```python
from build123d import *

# Parameters (mm, degrees)
SKETCH1_W           = 20
SKETCH1_H           = 20
BOSS_EXTRUDE1_DEPTH = 5
CHAMFER1_SIZE       = 3
FILLET1_R           = 3


with BuildPart() as part:
    # Sketch1 → Boss-Extrude1 (new body)
    with BuildSketch(Plane(origin=(0, 0, 0), x_dir=(1, 0, 0), z_dir=(0, 1, 0))):
        with Locations((10, 10)):
            Rectangle(SKETCH1_W, SKETCH1_H)
    extrude(amount=BOSS_EXTRUDE1_DEPTH)

    # Chamfer1
    chamfer1_edges = [part.edges().sort_by_distance(p)[0] for p in [
        (10, 5, -20),
        (0, 5, -10),
        (10, 5, 0),
        (20, 5, -10),
    ]]
    chamfer(chamfer1_edges, length=CHAMFER1_SIZE)

    # Fillet1
    # the kernel refuses this fillet: 3 mm, written as the material it takes off along each edge
    with BuildSketch(Plane(origin=(0, -7.5, 0), x_dir=(0, 0, -1), z_dir=(0, 1, 0)), Plane(origin=(0, -7.5, -20), x_dir=(1, 0, 0), z_dir=(0, 1, 0))) as fillet1_piece_1:
        with BuildLine():
            CenterArc((FILLET1_R, -FILLET1_R), FILLET1_R, 90, 90)
            Line((0, -FILLET1_R), (0, 0))
            Line((0, 0), (FILLET1_R, 0))
        make_face()
    extrude(amount=17, mode=Mode.SUBTRACT)
    with BuildSketch(Plane(origin=(20, -7.5, -20), x_dir=(-1, 0, 0), z_dir=(0, 1, 0)), Plane(origin=(20, -7.5, 0), x_dir=(0, 0, -1), z_dir=(0, 1, 0))) as fillet1_piece_2:
        with BuildLine():
            CenterArc((FILLET1_R, FILLET1_R), FILLET1_R, 180, 90)
            Line((0, FILLET1_R), (0, 0))
            Line((0, 0), (FILLET1_R, 0))
        make_face()
    extrude(amount=17, mode=Mode.SUBTRACT)
    with BuildSketch(Plane(origin=(22.5, -0.5, -22.5), x_dir=(-0.8164965809277263, -0.4082482904638636, -0.408248290463862), z_dir=(-0.5773502691896255, 0.577350269189626, 0.577350269189626)), Plane(origin=(22.5, -0.5, 2.5), x_dir=(0.4082482904638631, -0.4082482904638628, -0.8164965809277261), z_dir=(-0.5773502691896261, 0.5773502691896256, -0.5773502691896256))) as fillet1_piece_3:
        with BuildLine():
            CenterArc((FILLET1_R * 0.57735026919, FILLET1_R), FILLET1_R, 210, 60)
            Line((-FILLET1_R * 0.288675134595, FILLET1_R * 0.5), (0, 0))
            Line((0, 0), (FILLET1_R * 0.57735026919, 0))
        make_face()
    extrude(amount=13.856406461, mode=Mode.SUBTRACT)
    with BuildSketch(Plane(origin=(-2.5, -0.5, -22.5), x_dir=(0.8164965809277259, -0.40824829046386324, -0.40824829046386274), z_dir=(0.5773502691896258, 0.5773502691896258, 0.5773502691896258)), Plane(origin=(-2.5, -0.5, 2.5), x_dir=(-0.40824829046386274, -0.4082482904638633, -0.816496580927726), z_dir=(0.5773502691896258, 0.5773502691896258, -0.5773502691896258))) as fillet1_piece_4:
        with BuildLine():
            CenterArc((FILLET1_R * 0.57735026919, -FILLET1_R), FILLET1_R, 90, 60)
            Line((-FILLET1_R * 0.288675134595, -FILLET1_R * 0.5), (0, 0))
            Line((0, 0), (FILLET1_R * 0.57735026919, 0))
        make_face()
    extrude(amount=13.856406461, mode=Mode.SUBTRACT)


solid = part.part
```
Geometry: final body of the model. Coordinates: model frame, mm. Round coordinates to 2 decimals unless told otherwise and drop trailing zeros. Order: outer loops, then holes, each group sorted by start corner. A loop starts at its lowest first (then second) coordinate and runs counter-clockwise, first axis right, second up. Notation, with made-up numbers: M 42,86.5 L 50,86.5 A16 cw 50,108.5 Z; hole C 76.5,69 d4. An arc over 180 degrees is marked long. Use one line per item in the form item = value. Start each with the question number.
Q1. Cut plane A-A (x = 7.5). Return loops of the section in (y, z), and give its area (3 significant figures).
Q2. Material intervals for line 1 (Z direction, x = 2, y = 1.7); line 2 (X direction, y = 2.1, z = -7.25); line 3 (Z direction, x = 14.5, y = 4), sorted ascending. Write a range as [from, to].
Q3. Cut plane C-C (z = -6.5). Return loops of the section in (x, y).
Q4. Cut plane B-B (y = 1). Return loops of the section in (x, z).
Geometry results:
q1.outline = M 0,-20 L 2,-20 L 5,-17 L 5,-3 L 2,0 L 0,0 Z
q1.area = 91.0 mm^2
q2.line_1 = [-19.83, -0.17]
q2.line_2 = [0.1, 19.9]
q2.line_3 = [-18, -2]
q3.outline = M 0,0 L 20,0 L 20,2 L 17,5 L 3,5 L 0,2 Z
q4.outline = M 0,-17 A3 ccw 3,-20 L 17,-20 A3 ccw 20,-17 L 20,-3 A3 ccw 17,0 L 3,0 A3 ccw 0,-3 Z
